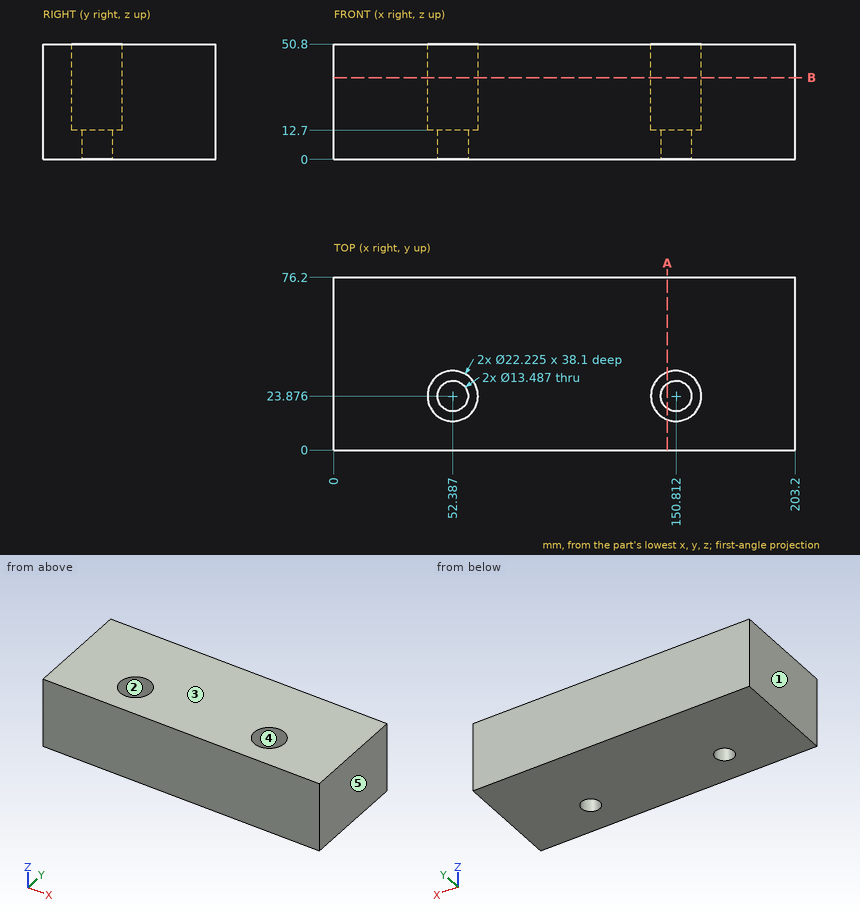
For this review, use the dimensioned drawing (mm, ordinates from the lowest corner) and the shaded views. A direction names the side the tool comes from. Round coordinates to 2 decimals unless told otherwise and drop trailing zeros. Write each loop counter-clockwise with the first axis right and the second up, starting at its lowest first coordinate (ties: lowest second). Pieces come first, ordered by that corner, then holes. Notation, with made-up numbers: M 53.5,33 L 96.5,33 A22 cw 96.5,46 Z; hole C 40,86 d5. An arc over 180 degrees is marked long. Use CSV: the item, a comma, the result in double quotes. Start each with the question number.
(1) Clearance check with a flat-ended pin moving along its axis: P1, Ø17.5, axis at x = 52.39, y = 23.88, coming from the +Z side. State where the tip first meets the part, or that it passes through.
(2) For line 1 along X through (y, z) = (21.5, 22.5); line 2 along X through (y, z) = (34, 44) (1 decimal); line 3 along Y through (x, z) = (160.5, 38.5) (1 decimal), list the stretches that pass through material, from the lowest coordinate up.
(3) We need section B-B, the plane z = 36. State the section outline as (x, y) points (1 decimal).
(4) Tool access review of the marked faces 1 and 2: name each direction out of +Z, -Z, +X, -X, +Y, -Y from which nothing blocks a thin tool from reaching the whole face with its end or side.
(5) We need section A-A, the plane x = 147. State the section outline as (y, z) points (1 decimal).
(6) The part is to be moulded in two halves that separate along X. For the marked faces 3, 4 and 5, say which applies: +X half, -X half, draft (parallel to the pull), parting line (faces both ways), or undercut.
Findings:
1,P1,"z = 12.7"
2,line 1,"0 to 41.53, 63.24 to 139.96, 161.67 to 203.2"
2,line 2,"0 to 47.8, 57 to 146.2, 155.4 to 203.2"
2,line 3,"0 to 18.4, 29.3 to 76.2"
3,outline,"M 0,0 L 203.2,0 L 203.2,76.2 L 0,76.2 Z; hole C 52.4,23.9 d22.2; hole C 150.8,23.9 d22.2"
4,face 1,"+Z, -Z, -X, +Y, -Y"
4,face 2,"+Z"
5,outline,"M 0,0 L 18.3,0 L 18.3,12.7 L 13.4,12.7 L 13.4,50.8 L 0,50.8 Z; M 29.4,0 L 76.2,0 L 76.2,50.8 L 34.3,50.8 L 34.3,12.7 L 29.4,12.7 Z"
6,face 3,"draft"
6,face 4,"undercut"
6,face 5,"+X half"
